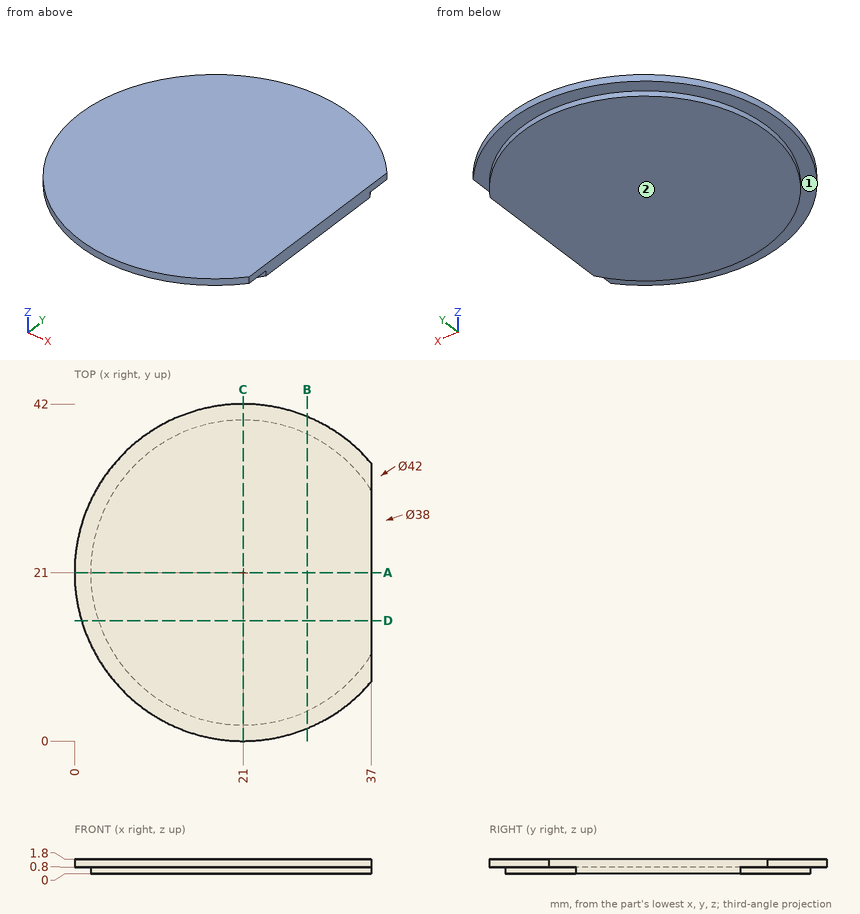
Geometry check sheet. Reference: drawing and pictorial views, mm from the part's lowest x, y, z. A direction names the side the tool comes from. Round coordinates to 2 decimals unless told otherwise and drop trailing zeros. Order: outer loops, then holes, each group sorted by start corner. A loop starts at its lowest first (then second) coordinate and runs counter-clockwise, first axis right, second up. Notation, with made-up numbers: M -39.5,87.5 L -30.5,87.5 A19 ccw -30.5,121.5 Z; hole C 3,60.5 d3. An arc over 180 degrees is marked long. Answer as CSV lines item,"result".
1) Gauge pin test, flat end, axial feed: pin 1 Ø1 at (y, z) = (35.5, 0.5) entering from -X. Record the tip position at first contact, or that the pin passes through.
Entries:
pin 1,"x = 5.44"
2) Sectioned sample at B-B on x = 29. Record the cut outline in (y, z).
Entries:
outline,"M 1.58,0.8 L 3.77,0.8 L 3.77,0 L 38.23,0 L 38.23,0.8 L 40.42,0.8 L 40.42,1.8 L 1.58,1.8 Z"
3) Thickness scan on probe 1 along Y at (x, z) = (21.5, 1.65); probe 2 along Y at (x, z) = (27, 1.1); probe 3 along Z at (x, y) = (5.5, 33). Record the ranges inside material, lowest first. Write a range as [from, to].
Entries:
probe 1,"[0.01, 41.99]"
probe 2,"[0.88, 41.12]"
probe 3,"[0.8, 1.8]"
4) Sectioned sample at A-A on y = 21. Record the cut outline in (x, z).
Entries:
outline,"M 0,0.8 L 2,0.8 L 2,0 L 37,0 L 37,1.8 L 0,1.8 Z"
5) Sectioned sample at C-C on x = 21. Record the cut outline in (y, z).
Entries:
outline,"M 0,0.8 L 2,0.8 L 2,0 L 40,0 L 40,0.8 L 42,0.8 L 42,1.8 L 0,1.8 Z"
6) Tool access check on the marked faces 1 and 2. Record the directions out of +Z, -Z, +X, -X, +Y, -Y that give a thin tool (end or side, any length) a straight path to the whole face; none if there is none.
Entries:
face 1,"-Z"
face 2,"-Z, +X, -X, +Y, -Y"
7) Sectioned sample at D-D on y = 15. Record the cut outline in (x, z).
Entries:
outline,"M 0.88,0.8 L 2.97,0.8 L 2.97,0 L 37,0 L 37,1.8 L 0.88,1.8 Z"
